For this review, take the finished solid that the model builds, in its own axes (mm). A direction names the side the tool comes from. Round coordinates to 2 decimals unless told otherwise and drop trailing zeros. Write each loop counter-clockwise with the first axis right and the second up, starting at its lowest first coordinate (ties: lowest second). Pieces come first, ordered by that corner, then holes. Notation, with made-up numbers: M 47.5,11 L 86.5,11 A25 cw 86.5,50 Z; hole C 37.25,14.25 d8. An arc over 180 degrees is marked long. Use one line per item in the form item = value. Start each with the question number.
Item 1: For line 1 (X direction, y = 0, z = 4.5); line 2 (X direction, y = 0, z = 9.5) (3 decimals); line 3 (Z direction, x = 23.55, y = -1.5), list the stretches that pass through material, from the lowest coordinate up. Write a range as [from, to].
Item 2: For P1, Ø3, axis at y = 1, z = 10, coming from the +X side; P2, Ø2.5, axis at x = 0, y = 0, coming from the -Z side; P3, Ø3, axis at y = -3, z = 2, coming from the -X side; P4, Ø1.8, axis at x = -1.5, y = -0.5, coming from the +Z side, all flat-tipped, find the tip position at first contact; note any pin that passes through.
Item 3: Add section D-D (y = -0.5). State the section outline as (x, z) points.
Item 4: Draft analysis for pull direction X (two halves, no side actions). For faces 6 (the flat face through (28, -4, 4.65)), 7 (the cylindrical face through (-6, 0, 6)), 8 (the flat face through (26, -3, 3.2)), state which applies: released by +X, released by -X, zero draft, split by the parting line, or undercut.
Item 5: Add section B-B (z = 1.5). State the section outline as (x, y) points, and give its area (3 significant figures).
Item 6: Add section C-C (x = -1). State the section outline as (y, z) points, and give its area (3 significant figures).
Item 7: Add section A-A (x = 25.5). State the section outline as (y, z) points.
Item 8: For faces 1 (the cylindrical face through (28.52, 0.15, 6.26)), 2 (the flat face through (32, 3, 6)), 3 (the flat face through (0, 2, 3.5)), 4 (the cylindrical face through (23.507, -1.715, 7.936)), 5 (the flat face through (25.479, 1.172, 7.872)), list the 3-axis set-ups (+Z, -Z, +X, -X, +Y, -Y) from which the entire face can be reached by the end or side of a thin tool; tool diameter is ignored.
Autodesk Fusion 360 part; units mm, degrees
sketch "Sketch1" plane through (0, 0, 0) normal (0, 0, 1) x (1, 0, 0)
  circle A0 centre (0, 0) radius 1.5
  line L0 (0, 6) -> (30, 6)
  line L1 (0, -6) -> (30, -6)
  arc A1 (0, 6) -> (0, -6) centre (0, 0) ccw
  line L2 (30, 6) -> (30, -6)
  dimension "d1" = 3
  dimension "d3" = 12
  dimension "d4" = 30
extrude "Extrude1" add sketch "Sketch1" along normal blind 12.6 makes body 1
sketch "Sketch2" plane through (30, 0, 0) normal (1, 0, 0) x (0, 1, 0)
  line L0 (-6, 0) -> (6, 0)
  line L1 (6, 0) -> (6, 12.6)
  line L2 (6, 12.6) -> (-6, 12.6)
  line L3 (-6, 12.6) -> (-6, 0)
  line L4 (6, 12.6) -> (3, 12.6)
  line L5 (3, 12.6) -> (3, 0)
  line L6 (3, 0) -> (6, 0)
  line L7 (6, 0) -> (6, 12.6)
  dimension "d7" = 3
extrude "Extrude2" add sketch "Sketch2" along normal blind 4.5 contours L0 L1 L2 L4 L5 L6 L7 bodies 1
ref_plane "WorkPlane1" through (14.25, 0, 6.3) normal (0, 0, 1) x (1, 0, 0)
ref_plane "WorkPlane2" through (15, 0, 6.3) normal (0, -1, 0) x (1, 0, 0)
sketch "Sketch3" plane through (0, -6, 0) normal (0, -1, 0) x (1, 0, 0)
  line L0 (0, 0) -> (30, 0)
  line L1 (30, 0) -> (30, 12.6)
  line L2 (30, 12.6) -> (0, 12.6)
  line L3 (0, 12.6) -> (0, 0)
  line L4 (13, 10.8) -> (24, 10.8)
  line L5 (24, 10.8) -> (24, 1.8)
  line L6 (24, 1.8) -> (13, 1.8)
  line L7 (13, 1.8) -> (13, 10.8)
  point P0 (30, 6.3)
  point P1 (24, 6.3)
  dimension "d15" = 9
  dimension "d16" = 11
  dimension "d17" = 6
sketch "Sketch6" plane through (0, -6, 0) normal (0, -1, 0) x (1, 0, 0)
  line L0 (0, 0) -> (30, 0)
  line L1 (30, 0) -> (30, 12.6)
  line L2 (30, 12.6) -> (0, 12.6)
  line L3 (0, 12.6) -> (0, 0)
  line L4 (24, 9.4) -> (27, 9.4)
  line L5 (27, 3.2) -> (24, 3.2)
  line L6 (24, 3.2) -> (24, 9.4)
  line L7 (27, 4.65) -> (30, 4.65)
  line L8 (30, 4.65) -> (30, 7.95)
  line L9 (30, 7.95) -> (27, 7.95)
  line L10 (27, 9.4) -> (27, 7.95)
  line L11 (27, 4.65) -> (27, 3.2)
  dimension "d28" = 3
  dimension "d29" = 3
  dimension "d30" = 3.3
  dimension "d39" = 6.2
ref_plane "WorkPlane3" through (15, -1.5, 6.3) normal (0, -1, 0) x (1, 0, 0)
extrude "Extrude6" cut sketch "Sketch6" against normal up to surface (4.5 mm away) contours L1 L4 L5 L6 L7 L8 L9 L10 L11 bodies 1
sketch "Sketch7" plane through (30, 0, 0) normal (1, 0, 0) x (0, 1, 0)
  line L0 (-6, 7.95) -> (-1.5, 7.95)
  line L1 (-1.5, 7.95) -> (-1.5, 4.65)
  line L2 (-1.5, 4.65) -> (-6, 4.65)
  line L3 (-6, 4.65) -> (-6, 0)
  line L4 (-6, 0) -> (3, 0)
  line L5 (3, 0) -> (3, 12.6)
  line L6 (3, 12.6) -> (-6, 12.6)
  line L7 (-6, 12.6) -> (-6, 7.95)
  circle A0 centre (-1.5, 6.3) radius 1.65
extrude "Extrude7" cut sketch "Sketch7" against normal blind 7 contours L1 A0 | L1 A0 bodies 1
sketch "Sketch8" plane through (24, 0, 0) normal (1, 0, 0) x (0, 1, 0)
  arc A0 (-1.5, 7.95) -> (-1.5, 4.65) centre (-1.5, 6.3) ccw
  line L0 (-1.5, 7.95) -> (-1.5, 9.4)
  line L1 (-1.5, 9.4) -> (-6, 9.4)
  line L2 (-6, 9.4) -> (-6, 3.2)
  line L3 (-6, 3.2) -> (-1.5, 3.2)
  line L4 (-1.5, 3.2) -> (-1.5, 4.65)
  line L5 (-3.2898, 9.4) -> (0.2898, 9.4)
  line L6 (0.2898, 9.4) -> (2.0796, 6.3)
  line L7 (2.0796, 6.3) -> (0.2898, 3.2)
  line L8 (0.2898, 3.2) -> (-3.2898, 3.2)
  line L9 (-3.2898, 3.2) -> (-5.0796, 6.3)
  line L10 (-5.0796, 6.3) -> (-3.2898, 9.4)
  line L11 (-1.5, 9.4) -> (-1.5, 3.2) construction
  point P0 (-1.5, 9.4)
  point P1 (-1.5, 3.2)
  point P2 (-1.5, 6.3)
  dimension "d36" = 120
extrude "Extrude8" cut sketch "Sketch8" along normal up to surface (3 mm away) contours A0 L0 L4 L5 L6 L7 L8 | A0 L0 L1 L3 L4 L5 L8 L9 L10 bodies 1
sketch "Sketch10" plane through (0, 0, 12.6) normal (0, 0, 1) x (-1, 0, 0)
  circle A0 centre (0, 0) radius 1.5
  arc A1 (0, -6) -> (0, 6) centre (0, 0) ccw
  line L0 (0, 6) -> (-30, 6)
  line L1 (-30, 6) -> (-30, -3)
  line L2 (-30, -3) -> (-34.5, -3)
  line L3 (-34.5, -3) -> (-34.5, -6)
  line L4 (-34.5, -6) -> (0, -6)
  circle A2 centre (0, 0) radius 2.945
  dimension "d40" = 5.89
extrude "Extrude9" cut sketch "Sketch10" against normal blind 7.1 contours A2 bodies 1
sketch "Sketch11" plane through (0, 0, 0) normal (0, 0, -1) x (1, 0, 0)
  circle A0 centre (0, 0) radius 1.5
  arc A1 (0, 6) -> (0, -6) centre (0, 0) ccw
  line L0 (0, -6) -> (34.5, -6)
  line L1 (34.5, -6) -> (34.5, -3)
  line L2 (34.5, -3) -> (30, -3)
  line L3 (30, -3) -> (30, 6)
  line L4 (30, 6) -> (0, 6)
  circle A2 centre (0, 0) radius 2.4
  dimension "d43" = 4.8
extrude "Extrude10" cut sketch "Sketch11" against normal blind 3.5 contours A2 bodies 1
copy_body "Body->Comp1" bodies 1 removing the originals makes body 2 in component "Component"
sketch "Sketch12" plane through (0, -6, 0) normal (0, -1, 0) x (1, 0, 0)
  line L0 (27, 7.95) -> (30, 7.95)
  line L1 (30, 7.95) -> (30, 12.6)
  line L2 (30, 12.6) -> (0, 12.6)
  line L3 (0, 12.6) -> (0, 0)
  line L4 (0, 0) -> (30, 0)
  line L5 (30, 0) -> (30, 4.65)
  line L6 (30, 4.65) -> (27, 4.65)
  line L7 (27, 4.65) -> (27, 3.2)
  line L8 (27, 3.2) -> (24.6, 3.2)
  line L9 (24.6, 3.2) -> (24.6, 9.4)
  line L10 (24.6, 9.4) -> (27, 9.4)
  line L11 (27, 9.4) -> (27, 7.95)
  line L12 (-8, 12.6) -> (20, 12.6)
  line L13 (20, 12.6) -> (20, 0)
  line L14 (20, 0) -> (-8, 0)
  line L15 (-8, 0) -> (-8, 12.6)
extrude "Extrude11" [suppressed]
component "Component" placed x (1, 0, 0) y (0, 1, 0) z (0, 0, 1) at (0, 0, 0)
Calculated:
q1.line_1 = [-6, -1.5], [1.5, 24], [27, 30]
q1.line_2 = [-6, -2.945], [2.945, 30]
q1.line_3 = [0, 4.65], [7.95, 12.6]
q2.P1 = 30
q2.P2 = through
q2.P3 = -5.81
q2.P4 = 5.5
q3.outline = M -5.98,0 L -2.35,0 L -2.35,3.5 L -1.41,3.5 L -1.41,5.5 L -2.9,5.5 L -2.9,12.6 L -5.98,12.6 Z; M 1.41,3.5 L 2.35,3.5 L 2.35,0 L 30,0 L 30,4.99 L 27,4.99 L 27,3.2 L 24,3.2 L 24,4.99 L 23,4.99 L 23,7.61 L 24,7.61 L 24,9.4 L 27,9.4 L 27,7.61 L 30,7.61 L 30,12.6 L 2.9,12.6 L 2.9,5.5 L 1.41,5.5 Z
q4.face_6 = zero draft
q4.face_7 = released by -X
q4.face_8 = undercut
q5.outline = M 0,-6 L 30,-6 L 30,3 L 34.5,3 L 34.5,6 L 0,6 A6 ccw Z; hole C 0,0 d4.8
q5.area = 412 mm^2
q6.outline = M -5.92,0 L -2.18,0 L -2.18,3.5 L -1.12,3.5 L -1.12,5.5 L -2.77,5.5 L -2.77,12.6 L -5.92,12.6 Z; M 1.12,3.5 L 2.18,3.5 L 2.18,0 L 5.92,0 L 5.92,12.6 L 2.77,12.6 L 2.77,5.5 L 1.12,5.5 Z
q6.area = 90.0 mm^2
q7.outline = M -6,0 L 6,0 L 6,12.6 L -6,12.6 L -6,9.4 L 0.29,9.4 L 2.08,6.3 L 0.29,3.2 L -6,3.2 Z
q8.face_1 = +X, -Y
q8.face_2 = +Z, -Z, +X, -Y
q8.face_3 = -Z
q8.face_4 = +X
q8.face_5 = -Y
